For this review, take the finished solid that the model builds, in its own axes (mm). Coordinates: 2 decimals unless noted, no trailing zeros. Order: outer loops, then holes, each group sorted by start corner. A loop starts at its lowest first (then second) coordinate and runs counter-clockwise, first axis right, second up. Notation, with made-up numbers: (-10.75, 24.25) -> (26.25, 24.25) arc R26 ccw to (26.25, 62.25) -> close; hole circle Ø10 at (27, -26.5). An arc over 180 degrees is marked (long way). Answer as a JSON object with one key per item and string values. Group by question number.
1) Add section A-A, the plane y = 0. Write out the cut boundary in (x, z).
2) Add section D-D, the plane y = 110.5. Write out the cut boundary in (x, z), then the cut area to 3 significant figures.
3) Wall thickness on L1, parallel to Y at x = -3, z = 1.1; L2, parallel to X at y = 31, z = 4.5; L3, parallel to X at y = 72, z = 4.65: over which ranges is each line inside the solid? List them lowest first.
4) Draft analysis for pull direction X (two halves, no side actions). For faces 1 (the cylindrical face through (-2.4, 128.64, 2.54)), 2 (the cylindrical face through (-2.4, 120.95, 2.54)), 3 (the flat face through (-7, 51, 0)), 4 (the cylindrical face through (2.795, -12.184, 2.465)), state which applies: +X half, -X half, draft (parallel to the pull), parting line (faces both ways), or undercut.
5) Add section B-B, the plane z = 2.5. Count the separate pieces of the cut face and the enclosed holes in it, then the cut area to 3 significant figures.
6) For pin 1 (2.5 mm diameter, centred on x = -2.3, y = 12.06, fed in from -Z); pin 2 (4.5 mm diameter, centred on x = -1.96, y = 130.64, fed in from -Z); pin 3 (1 mm diameter, centred on x = 0.5, z = 2, fed in from +Y), all flat-tipped, find the tip position at first contact; note any pin that passes through.
from build123d import *

# Parameters (mm, degrees)
SCHIZZO1_R                   = 2.05
ESTRUSIONE_ESTRUSIONE1_DEPTH = 5
TAGLIO_ESTRUSIONE1_REACH     = 7
SCHIZZO2_R                   = 2.05
SKETCH1_R                    = 2.05
CUT_EXTRUDE1_DEPTH           = 5
CUT_EXTRUDE2_REACH           = 7
SKETCH2_R                    = 2.05


with BuildPart() as part:
    # Schizzo1 → Estrusione-Estrusione1 (new body)
    with BuildSketch(Plane.XY):
        with BuildLine():
            ThreePointArc((7.023974797, 138.427683332), (1.499753731, 147.278176914), (-7.525391936, 142.044153534))
            ThreePointArc((-7.525391936, 142.044153534), (-18.729107246, 69.99949188), (-12.22229981, -2.620188418))
            ThreePointArc((-12.22229981, -2.620188418), (3.068449146, -12.117533571), (11.996332959, 3.512548298))
            ThreePointArc((11.996332959, 3.512548298), (1.102237583, 70.660238267), (7.023974797, 138.427683332))
        make_face()
        Circle(SCHIZZO1_R, mode=Mode.SUBTRACT)
        with Locations((-0.309434746, 139.999658036)):
            Circle(SCHIZZO1_R, mode=Mode.SUBTRACT)
    extrude(amount=ESTRUSIONE_ESTRUSIONE1_DEPTH)

    # Schizzo2 → Taglio-Estrusione1 (cut, up to next)
    with BuildSketch(Plane.XY.offset(5), mode=Mode.PRIVATE) as taglio_estrusione1_sk1:
        with Locations((-6.142115432, 104.166670735)):
            Circle(SCHIZZO2_R)
    taglio_estrusione1_tool1 = extrude(taglio_estrusione1_sk1.sketch, amount=-TAGLIO_ESTRUSIONE1_REACH, mode=Mode.PRIVATE) & part.part
    add(taglio_estrusione1_tool1.solids().sort_by_distance((-6.142115, 104.166671, 5))[0], mode=Mode.SUBTRACT)
    # Schizzo2 → Taglio-Estrusione1 (cut, up to next)
    with BuildSketch(Plane.XY.offset(5), mode=Mode.PRIVATE) as taglio_estrusione1_sk2:
        with Locations((-6.142115432, 32.213749463)):
            Circle(SCHIZZO2_R)
    taglio_estrusione1_tool2 = extrude(taglio_estrusione1_sk2.sketch, amount=-TAGLIO_ESTRUSIONE1_REACH, mode=Mode.PRIVATE) & part.part
    add(taglio_estrusione1_tool2.solids().sort_by_distance((-6.142115, 32.213749, 5))[0], mode=Mode.SUBTRACT)

    # Sketch1 → Cut-Extrude1 (cut)
    with BuildSketch(Plane.XY.offset(5)):
        with Locations((-0.309434746, 139.999658036)):
            Circle(SKETCH1_R)
        with Locations((-1.959092434, 130.643984382)):
            Circle(SKETCH1_R)
        with Locations((-3.348277855, 122.765522358)):
            Circle(SKETCH1_R)
    extrude(amount=-CUT_EXTRUDE1_DEPTH, mode=Mode.SUBTRACT)

    # Sketch2 → Cut-Extrude2 (cut, up to next)
    with BuildSketch(Plane.XY.offset(5), mode=Mode.PRIVATE) as cut_extrude2_sk1:
        with Locations((-0.872956087, 4.578420741)):
            Circle(SKETCH2_R)
    cut_extrude2_tool1 = extrude(cut_extrude2_sk1.sketch, amount=-CUT_EXTRUDE2_REACH, mode=Mode.PRIVATE) & part.part
    add(cut_extrude2_tool1.solids().sort_by_distance((-0.872956, 4.578421, 5))[0], mode=Mode.SUBTRACT)
    # Sketch2 → Cut-Extrude2 (cut, up to next)
    with BuildSketch(Plane.XY.offset(5), mode=Mode.PRIVATE) as cut_extrude2_sk2:
        with Locations((-2.300132251, 12.063577265)):
            Circle(SKETCH2_R)
    cut_extrude2_tool2 = extrude(cut_extrude2_sk2.sketch, amount=-CUT_EXTRUDE2_REACH, mode=Mode.PRIVATE) & part.part
    add(cut_extrude2_tool2.solids().sort_by_distance((-2.300132, 12.063577, 5))[0], mode=Mode.SUBTRACT)


solid = part.part
Output values:
{
 "1": {"outline": "(-12.77, 0) -> (-2.05, 0) -> (-2.05, 5) -> (-12.77, 5) -> close; (2.05, 0) -> (12.5, 0) -> (12.5, 5) -> (2.05, 5) -> close"},
 "2": {"outline": "(-14.65, 0) -> (2.53, 0) -> (2.53, 5) -> (-14.65, 5) -> close", "area": "85.9 mm²"},
 "3": {"L1": "y = -12.13 to 10.14, 13.99 to 120.75, 124.79 to 128.88, 132.41 to 147", "L2": "x = -17.46 to -7.79, -4.49 to 5.46", "L3": "x = -18.66 to 1.06"},
 "4": {"face 1": "undercut", "face 2": "undercut", "face 3": "draft", "face 4": "parting line"},
 "5": {"separate pieces": "1", "enclosed holes": "8", "area": "3,040 mm²"},
 "6": {"pin 1": "passes through", "pin 2": "stops at z = 0", "pin 3": "stops at y = 147.49"}
}
